```python
from build123d import *

# Parameters (mm, degrees)
F2_W          = 40
F2_H          = 60
F3_DEPTH      = 3
F5_DEPTH      = 15
F5_DEPTH_BACK = 15
F7_DEPTH      = 30
F8_R          = 1.5


with BuildPart() as f3:
    # F2 (on Top) → F3 (new body)
    with BuildSketch(Plane.XY):
        with Locations((0, 30)):
            Rectangle(F2_W, F2_H)
    extrude(amount=F3_DEPTH)

    # F4 (on Right) → F5 (join, two sides)
    with BuildSketch(Plane.YZ) as f5_sk:
        Polygon((60, 3), (60, 13.5796188425), (0, 3), align=None)
    extrude(amount=F5_DEPTH)
    extrude(f5_sk.sketch, amount=-F5_DEPTH_BACK)

    # F6 (on face) → F7 (cut, through all)
    with BuildSketch(Plane.YZ.offset(15)):
        Polygon((17.2763114494, 3), (57, 3), (57, 10.0043580647), align=None)
    extrude(amount=-F7_DEPTH, mode=Mode.SUBTRACT)

    # F8
    f8_edges = [f3.edges().sort_by_distance(p)[0] for p in [
        (0, 57, 3),
        (0, 57, 10.004358),
        (0, 17.276311, 3),
    ]]
    fillet(f8_edges, radius=F8_R)


solid = f3.part
```
CAD build for the part. Positions are in the model's coordinates, mm. A direction names the side the tool comes from. Coordinates: 2 decimals unless noted, no trailing zeros. Write each loop counter-clockwise with the first axis right and the second up, starting at its lowest first coordinate (ties: lowest second). Pieces come first, ordered by that corner, then holes.
(1) Cut at A-A, the plane x = -8. List the corners of the cut face in (y, z).
(2) Drill centre lines: probe 1 along X at (y, z) = (23.5, 5); probe 2 along Z at (x, y) = (-11, 53); probe 3 along Z at (x, y) = (15.5, 53.5). Where is each one in solid material? Low to high.
(3) Two-plate mould, pull along Y, no slides. Class faces 1 (the face through (-15, 37, 7)), 2 (the face through (0.21, 30.42, 8.364)), 3 (the face through (0, 57, 6)), 4 (the face through (0.21, 44.85, 7.86)): +Y half, -Y half, draft (parallel to the pull), parting line (faces both ways), or undercut.
(4) Cut at D-D, the plane z = 12.75. List the corners of the cut face in (x, y) (3 decimals).
(5) 3-axis set-ups, long thin cutter, end or side, ignore diameter. For faces 5 (the face through (15, 37, 7)), 6 (the face through (0, 37, 3)), 7 (the face through (-0.21, 56.55, 3.43)): which of +Z, -Z, +X, -X, +Y, -Y reach the whole face in a straight line?
(6) Flat gauge pins, fed straight in: pin 1 (6 mm diameter, centred on x = 2, y = 16, fed in from +Z); pin 2 (12 mm diameter, centred on x = -12.5, y = 17, fed in from +Z); pin 3 (1 mm diameter, centred on x = 2.5, y = 38, fed in from +Z). Where does each tip first touch, or does it go through?
(7) Cut at B-B, the plane y = 52.5. List the corners of the cut face in (x, z), and give its area (3 significant figures).
(8) Cut at C-C, the plane y = 14.5. List the corners of the cut face in (x, z).
Geometry says:
1. outline: (0, 0) - (60, 0) - (60, 13.58) - (0, 3) - close; hole (34.16, 5.98) arc R1.5 ccw to (34.42, 3) - (55.5, 3) arc R1.5 ccw to (57, 4.5) - (57, 8.22) arc R1.5 ccw to (55.24, 9.69) - close
2. probe 1: x = -15 to 15
2. probe 2: z = 0 to 3, 9.3 to 12.35
2. probe 3: z = 0 to 3
3. face 1: draft
3. face 2: -Y half
3. face 3: undercut
3. face 4: undercut
4. outline: (-15, 55.295) - (15, 55.295) - (15, 60) - (-15, 60) - close
5. face 5: +Z, +X, +Y, -Y
5. face 6: none
5. face 7: +X, -X
6. pin 1: stops at z = 6.35
6. pin 2: stops at z = 7.06
6. pin 3: stops at z = 9.79
7. outline: (-20, 0) - (20, 0) - (20, 3) - (-20, 3) - close; (-15, 9.21) - (15, 9.21) - (15, 12.26) - (-15, 12.26) - close
7. area: 211 mm2
8. outline: (-20, 0) - (20, 0) - (20, 3) - (15, 3) - (15, 5.56) - (-15, 5.56) - (-15, 3) - (-20, 3) - close
